Part model, mm, in its own coordinate system. A direction names the side the tool comes from. Round coordinates to 2 decimals unless told otherwise and drop trailing zeros. Loops run counter-clockwise (first coordinate to the right, second up) from the corner with the lowest first, then second, coordinate; pieces in that order, holes last. Notation, with made-up numbers: M -18,10 L -4,10 A13 cw -4,16 Z; hole C 41.25,-8 d1. An arc over 180 degrees is marked long. Write each question's results on one line, items separated by ' | '.
from build123d import *

# Parameters (mm, degrees)
SKETCH1_R           = 5
SKETCH1_R_2         = 3
BOSS_EXTRUDE1_DEPTH = 7
SKETCH2_R           = 3
BOSS_EXTRUDE2_DEPTH = 7
SKETCH3_W           = 16.288395929
SKETCH3_H           = 13.1
BOSS_EXTRUDE3_DEPTH = 4
SKETCH4_W           = 4.517614974
SKETCH4_H           = 7
CUT_EXTRUDE1_DEPTH  = 4
BOSS_EXTRUDE4_DEPTH = 4
BOSS_EXTRUDE5_DEPTH = 4
BOSS_EXTRUDE6_DEPTH = 19
BOSS_EXTRUDE7_DEPTH = 4
BOSS_EXTRUDE8_DEPTH = 8.1
SKETCH10_W          = 12.1
SKETCH10_H          = 15.357517161
CUT_EXTRUDE2_DEPTH  = 90.333377092
CUT_EXTRUDE3_DEPTH  = 87.16880235
SKETCH12_W          = 10.311784895
SKETCH12_H          = 4.86074743
CUT_EXTRUDE4_DEPTH  = 10


with BuildPart() as part:
    # Sketch1 → Boss-Extrude1 (new body)
    with BuildSketch(Plane(origin=(0, 0, 0), x_dir=(1, 0, 0), z_dir=(0, 1, 0))):
        with Locations(Location((0, 0, 0), (0, 0, 270))):
            Circle(SKETCH1_R)
        with Locations(Location((0, 0, 0), (0, 0, 270))):
            Circle(SKETCH1_R_2, mode=Mode.SUBTRACT)
    extrude(amount=BOSS_EXTRUDE1_DEPTH)

    # Sketch2 → Boss-Extrude2 (add, through all)
    with BuildSketch(Plane(origin=(0, 7, 0), x_dir=(1, 0, 0), z_dir=(0, 1, 0))):
        with BuildLine():
            Line((4.582575695, -2), (34.582575695, -2))
            Line((34.582575695, -2), (34.582575695, 2))
            Line((34.582575695, 2), (4.582575695, 2))
            ThreePointArc((4.582575695, 2), (-5, 0), (4.582575695, -2))
        make_face()
        with Locations(Location((0, 0, 0), (0, 0, 270))):
            Circle(SKETCH2_R, mode=Mode.SUBTRACT)
    extrude(amount=-BOSS_EXTRUDE2_DEPTH)

    # Sketch3 → Boss-Extrude3 (add)
    with BuildSketch(Plane.XY.offset(2)):
        with Locations((21.920762757, 6.55)):
            Rectangle(SKETCH3_W, SKETCH3_H)
    extrude(amount=-BOSS_EXTRUDE3_DEPTH)

    # Sketch4 → Cut-Extrude1 (cut)
    with BuildSketch(Plane.XY.offset(2)):
        with Locations((32.323768208, 3.5)):
            Rectangle(SKETCH4_W, SKETCH4_H)
    extrude(amount=-CUT_EXTRUDE1_DEPTH, mode=Mode.SUBTRACT)

    # Sketch5 → Boss-Extrude4 (add)
    with BuildSketch(Plane.XY.offset(2)):
        Polygon((30.064960721, 13.1), (30.064960721, 0), (36.964960721, 0), (50.064960721, 13.1), (76.225581431, 13.1), (80.064960721, 19.75), (80.064960721, 26.4), (43.364960721, 26.4), align=None)
    extrude(amount=-BOSS_EXTRUDE4_DEPTH)

    # Sketch6 → Boss-Extrude5 (add)
    with BuildSketch(Plane.XY.offset(2)):
        Polygon((64.244452646, 36.204482672), (68.244452646, 36.204482672), (49.244452646, 3.295517328), (45.244452646, 3.295517328), align=None)
        Polygon((85.564960721, 36.204482672), (89.564960721, 36.204482672), (70.564960721, 3.295517328), (66.564960721, 3.295517328), align=None)
    extrude(amount=-BOSS_EXTRUDE5_DEPTH)

    # Sketch7 → Boss-Extrude6 (add)
    with BuildSketch(Plane.XY.offset(2)):
        Polygon((68.244452646, 36.204482672), (64.244452646, 36.204482672), (61.935051569, 32.204482672), (65.935051569, 32.204482672), align=None)
        Polygon((85.564960721, 36.204482672), (89.564960721, 36.204482672), (87.255559645, 32.204482672), (83.255559645, 32.204482672), align=None)
        Polygon((66.564960721, 3.295517328), (70.564960721, 3.295517328), (72.874361798, 7.295517328), (68.874361798, 7.295517328), align=None)
        Polygon((45.244452646, 3.295517328), (49.244452646, 3.295517328), (51.553853723, 7.295517328), (47.553853723, 7.295517328), align=None)
    extrude(amount=BOSS_EXTRUDE6_DEPTH)

    # Sketch8 → Boss-Extrude7 (add)
    with BuildSketch(Plane.XY.offset(21)):
        Polygon((64.244452646, 36.204482672), (68.244452646, 36.204482672), (49.244452646, 3.295517328), (45.244452646, 3.295517328), align=None)
        Polygon((85.564960721, 36.204482672), (89.564960721, 36.204482672), (70.564960721, 3.295517328), (66.564960721, 3.295517328), align=None)
    extrude(amount=-BOSS_EXTRUDE7_DEPTH)

    # Sketch9 → Boss-Extrude8 (add)
    with BuildSketch(Plane(origin=(0, 0, -2), x_dir=(-1, 0, 0), z_dir=(0, 0, -1))):
        Polygon((-54.905073356, 13.1), (-62.583831936, 26.4), (-83.95273694, 26.483825938), (-76.273978359, 13.183825938), align=None)
    extrude(amount=BOSS_EXTRUDE8_DEPTH)

    # Sketch10 → Cut-Extrude2 (cut, through all)
    with BuildSketch(Plane(origin=(51.496719679, -29.731644969, 0), x_dir=(0, 0, -1), z_dir=(0.8660254037844388, -0.49999999999999983, 0))):
        with Locations((4.05, 57.233275941)):
            Rectangle(SKETCH10_W, SKETCH10_H)
    extrude(amount=-CUT_EXTRUDE2_DEPTH, mode=Mode.SUBTRACT)

    # Sketch11 → Cut-Extrude3 (cut, through all)
    with BuildSketch(Plane(origin=(48.496719679, -27.999594161, 0), x_dir=(0, 0, 1), z_dir=(-0.8660254037844388, 0.49999999999999983, 0))):
        Polygon((-20.134561074, 86.736839969), (39.285177729, 86.736839969), (39.285177729, 23.813896611), (39.285177729, -9.631836795), (-20.134561074, -9.631836795), (-20.134561074, 23.813896611), align=None)
    extrude(amount=CUT_EXTRUDE3_DEPTH, mode=Mode.SUBTRACT)

    # Sketch12 → Cut-Extrude4 (cut)
    with BuildSketch(Plane(origin=(51.496719679, -29.731644969, 0), x_dir=(0, 0, -1), z_dir=(0.8660254037844388, -0.49999999999999983, 0))):
        with Locations((7.155892448, 47.124143646)):
            Rectangle(SKETCH12_W, SKETCH12_H)
    extrude(amount=-CUT_EXTRUDE4_DEPTH, mode=Mode.SUBTRACT)


solid = part.part
Item 1: Band-saw the part on C-C on y = 23. Give the cut face in (x, z), and give its area (3 significant figures).
Filled sheet:
outline: M 77.94,17 L 81.94,17 L 81.94,21 L 77.94,21 Z | area: 16.0 mm^2
Item 2: Wall check: L1, parallel to Z at x = 75.5, y = 16; L2, parallel to Y at x = 86.5, z = 7.25; L3, parallel to Z at x = 70.5, y = 8. Give the ranges that are in metal, low to high.
Filled sheet:
L1: 17 to 21 | L2: 32.2 to 36.2 | L3: -2 to 2, 17 to 21
Item 3: Which spindle directions (+Z, -Z, +X, -X, +Y, -Y) get a long thin tool onto all of the face, cutting with end or side? Do faces 4 (the flat face through (71, 7.296, 9)), 5 (the flat face through (84, 30, 2)), 6 (the flat face through (74.79, 14.04, 0.03)), 7 (the flat face through (82.47, 27.34, 0.03)), 8 (the flat face through (78, 20, 17)). Say none if no direction does.
Filled sheet:
face 4: +X, -X, +Y | face 5: +X, -X, -Y | face 6: -Z, +X, +Y | face 7: -Z, -X, -Y | face 8: +X, -X
Item 4: Band-saw the part on B-B on z = 15.75. Give the cut face in (x, y).
Filled sheet:
outline: M 66.56,3.3 L 70.56,3.3 L 72.87,7.3 L 68.87,7.3 Z; M 83.26,32.2 L 87.26,32.2 L 89.56,36.2 L 85.56,36.2 Z
Item 5: Drop flat-ended pins along their axis: P1, Ø3, axis at y = 17.5, z = 16, coming from the -X side; P2, Ø3, axis at y = 33, z = 7.5, coming from the +X side; P3, Ø2, axis at x = 74.5, z = 17, coming from the +Y side. Give the stop position or say it passes through.
Filled sheet:
P1: x = 74.12 | P2: x = 88.58 | P3: y = 18.77
Item 6: Two-plate mould, pull along Z, no slides. Class faces 1 (the flat face through (78, 21, 21)), 2 (the flat face through (69, 3.296, 10)), 3 (the flat face through (73, 11, 2)): +Z half, -Z half, draft (parallel to the pull), parting line (faces both ways), or undercut.
Filled sheet:
face 1: +Z half | face 2: draft | face 3: undercut
Item 7: Band-saw the part on A-A on x = 81.5. Give the cut face in (y, z).
Filled sheet:
outline: M 22.24,17 L 29.16,17 L 29.16,21 L 22.24,21 Z; M 27.9,-2 L 29.16,-2 L 29.16,2 L 27.9,2 Z
